Geometry check sheet. Reference: the model listing, model coordinates, mm. Give positions to 0.01 mm unless a question says otherwise; leave off trailing zeros. Write each loop counter-clockwise with the first axis right and the second up, starting at its lowest first coordinate (ties: lowest second). Pieces come first, ordered by that corner, then holes. Notation, with made-up numbers: M -12,29.5 L 1,29.5 A12 ccw 1,45.5 Z; hole C 5.5,-37 d11. An arc over 180 degrees is marked long. Use one line per item in the form item = value. Start each with the question number.
```python
from build123d import *

# Parameters (mm, degrees)
F0_W     = 50
F0_H     = 50
F1_DEPTH = 40
F2_W     = 10
F2_H     = 10
F3_DEPTH = 80
F4_R     = 2.5
F5_R     = 2.5
F6_R     = 2.5
F7_R     = 2.5
F8_R     = 5
F9_R     = 5


with BuildPart() as f1:
    # F0 (on Top) → F1 (new body)
    with BuildSketch(Plane.XY):
        Rectangle(F0_W, F0_H)
    extrude(amount=F1_DEPTH)

    # F2 (on face) → F3 (join)
    with BuildSketch(Plane.YZ.offset(25)):
        with Locations((0, 17.170411)):
            Rectangle(F2_W, F2_H)
    extrude(amount=F3_DEPTH)

    # F4
    f4_edges = [f1.edges().sort_by_distance(p)[0] for p in [
        (65, 5, 22.170411),
    ]]
    fillet(f4_edges, radius=F4_R)

    # F5
    f5_edges = [f1.edges().sort_by_distance(p)[0] for p in [
        (65, -5, 22.170411),
    ]]
    fillet(f5_edges, radius=F5_R)

    # F6
    f6_edges = [f1.edges().sort_by_distance(p)[0] for p in [
        (65, -5, 12.170411),
    ]]
    fillet(f6_edges, radius=F6_R)

    # F7
    f7_edges = [f1.edges().sort_by_distance(p)[0] for p in [
        (65, 5, 12.170411),
    ]]
    fillet(f7_edges, radius=F7_R)

    # F8
    f8_edges = [f1.edges().sort_by_distance(p)[0] for p in [
        (0, 25, 40),
    ]]
    fillet(f8_edges, radius=F8_R)

    # F9
    f9_edges = [f1.edges().sort_by_distance(p)[0] for p in [
        (0, -25, 40),
    ]]
    fillet(f9_edges, radius=F9_R)


solid = f1.part
```
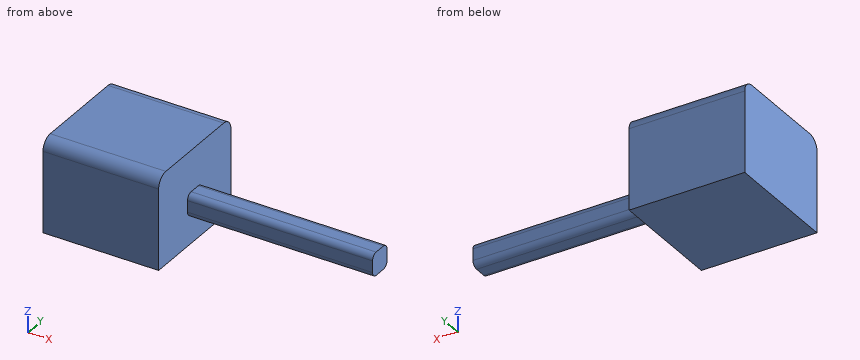
(1) Depth check by flat-ended pin: pin 1 (2.5 mm diameter, centred on x = 67.5, y = 0.5, fed in from +Z); pin 2 (12 mm diameter, centred on y = -12, z = 16.5, fed in from +X); pin 3 (1 mm diameter, centred on x = 42.5, z = 18, fed in from +Y). Enter the tip coordinate at first touch or a pass-through.
(2) Sectioned sample at D-D, the plane y = -12.5. Record the boundary of the cut face in (x, z).
(3) Sectioned sample at C-C, the plane z = 27.5. Record the boundary of the cut face in (x, y), plus the area to 3 significant figures.
(4) Sectioned sample at B-B, the plane x = 28.5. Record the boundary of the cut face in (y, z).
(5) Sectioned sample at A-A, the plane y = 0. Record the boundary of the cut face in (x, z).
(6) Thickness scan on probe 1 along X at (y, z) = (21.5, 36); probe 2 along Z at (x, y) = (71.5, -1.5); probe 3 along Y at (x, z) = (85, 19). Record the ranges inside material, lowest first. Write a range as [from, to].
Numbers:
q1.pin_1 = 22.17
q1.pin_2 = 25
q1.pin_3 = 5
q2.outline = M -25,0 L 25,0 L 25,40 L -25,40 Z
q3.outline = M -25,-25 L 25,-25 L 25,25 L -25,25 Z
q3.area = 2,500 mm2
q4.outline = M -5,14.67 A2.5 ccw -2.5,12.17 L 2.5,12.17 A2.5 ccw 5,14.67 L 5,19.67 A2.5 ccw 2.5,22.17 L -2.5,22.17 A2.5 ccw -5,19.67 Z
q5.outline = M -25,0 L 25,0 L 25,12.17 L 105,12.17 L 105,22.17 L 25,22.17 L 25,40 L -25,40 Z
q6.probe_1 = [-25, 25]
q6.probe_2 = [12.17, 22.17]
q6.probe_3 = [-5, 5]
